Geometry: final body of the model. Coordinates: model frame, mm. Coordinates: 2 decimals unless noted, no trailing zeros. Order: outer loops, then holes, each group sorted by start corner. A loop starts at its lowest first (then second) coordinate and runs counter-clockwise, first axis right, second up. Notation, with made-up numbers: M -21.5,-3 L 14.5,-3 A16 ccw 14.5,26 Z; hole C 27.25,38 d4. An arc over 180 degrees is marked long. Write item = value, one per line.
from build123d import *

# Parameters (mm, degrees)
EXTRUDE_1_DEPTH     = 3
SKETCH_3_R          = 1.6
CUT_EXTRUDE_1_DEPTH = 92.836811791


with BuildPart() as part:
    # 草图1 → 凸台-拉伸1 (new body)
    with BuildSketch(Plane.XY):
        Polygon((0, 0), (0, 15), (13, 15), (30, 32), (30, 45), (50, 45), (50, 32), (67, 15), (80, 15), (80, 0), align=None)
    extrude(amount=EXTRUDE_1_DEPTH)

    # 草图3 → 切除-拉伸1 (cut, through all)
    with BuildSketch(Plane(origin=(0, 0, 0), x_dir=(-1, 0, 0), z_dir=(0, 0, -1))):
        with Locations((-46, 41)):
            Circle(SKETCH_3_R)
        with Locations((-34, 41)):
            Circle(SKETCH_3_R)
        with Locations((-46, 19)):
            Circle(SKETCH_3_R)
        with Locations((-34, 19)):
            Circle(SKETCH_3_R)
        with Locations((-34, 30)):
            Circle(SKETCH_3_R)
        with Locations((-46, 30)):
            Circle(SKETCH_3_R)
        with Locations((-74, 7)):
            Circle(SKETCH_3_R)
        with Locations((-66, 7)):
            Circle(SKETCH_3_R)
        with Locations((-58, 7)):
            Circle(SKETCH_3_R)
        with Locations((-50, 7)):
            Circle(SKETCH_3_R)
        with Locations((-6, 7)):
            Circle(SKETCH_3_R)
        with Locations((-14, 7)):
            Circle(SKETCH_3_R)
        with Locations((-22, 7)):
            Circle(SKETCH_3_R)
        with Locations((-29, 7)):
            Circle(SKETCH_3_R)
        with BuildLine():
            Line((-61.292893219, 16.464466094), (-55.636038969, 22.121320344))
            ThreePointArc((-55.636038969, 22.121320344), (-51.393398282, 22.121320344), (-51.393398282, 17.878679656))
            Line((-51.393398282, 17.878679656), (-57.050252532, 12.221825407))
            ThreePointArc((-57.050252532, 12.221825407), (-61.292893219, 12.221825407), (-61.292893219, 16.464466094))
        make_face()
        with BuildLine():
            Line((-22.949747468, 12.221825407), (-28.606601718, 17.878679656))
            ThreePointArc((-28.606601718, 17.878679656), (-28.606601718, 22.121320344), (-24.363961031, 22.121320344))
            Line((-24.363961031, 22.121320344), (-18.707106781, 16.464466094))
            ThreePointArc((-18.707106781, 16.464466094), (-18.707106781, 12.221825407), (-22.949747468, 12.221825407))
        make_face()
        with BuildLine():
            Line((-43, 5), (-43, 13))
            ThreePointArc((-43, 13), (-40, 16), (-37, 13))
            Line((-37, 13), (-37, 5))
            ThreePointArc((-37, 5), (-40, 2), (-43, 5))
        make_face()
    extrude(amount=-CUT_EXTRUDE_1_DEPTH, mode=Mode.SUBTRACT)


solid = part.part
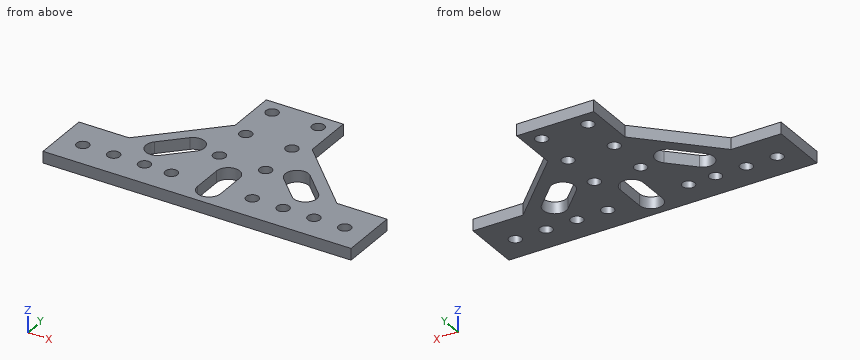
1) Line query: L1, parallel to Y at x = 46, z = 2; L2, parallel to Y at x = 40, z = 2.4; L3, parallel to X at y = 16.5, z = 0.3. Output: solid intervals per line, ascending.
Numbers:
L1 = 0 to 17.4, 20.6 to 28.4, 31.6 to 39.4, 42.6 to 45
L2 = 0 to 2, 16 to 45
L3 = 14.5 to 18.74, 27.23 to 52.77, 61.26 to 65.5
2) Section C-C, the plane x = 22. Return loops of the section in (y, z), and give its area (3 significant figures).
Numbers:
outline = M 0,0 L 5.4,0 L 5.4,3 L 0,3 Z; M 8.6,0 L 11.58,0 L 11.58,3 L 8.6,3 Z; M 19.76,0 L 24,0 L 24,3 L 19.76,3 Z
area = 37.9 mm²
3) Section A-A, the plane y = 41. Return loops of the section in (x, z), and give its area (3 significant figures).
Numbers:
outline = M 30,0 L 32.4,0 L 32.4,3 L 30,3 Z; M 35.6,0 L 44.4,0 L 44.4,3 L 35.6,3 Z; M 47.6,0 L 50,0 L 50,3 L 47.6,3 Z
area = 40.8 mm²
4) Section B-B, the plane x = 6. Return loops of the section in (y, z).
Numbers:
outline = M 0,0 L 5.4,0 L 5.4,3 L 0,3 Z; M 8.6,0 L 15,0 L 15,3 L 8.6,3 Z
5) Section D-D, the plane x = 14. Return loops of the section in (y, z), and give its area (3 significant figures).
Numbers:
outline = M 0,0 L 5.4,0 L 5.4,3 L 0,3 Z; M 8.6,0 L 16,0 L 16,3 L 8.6,3 Z
area = 38.4 mm²
6) Pin query (flat end, axial travel): pin 1 (3 mm diameter, centred on x = 50, y = 7, fed in from +Z); pin 2 (3.5 mm diameter, centred on x = 22, y = 7, fed in from +Z). Return the tip coordinate at first contact, or that it passes through.
Numbers:
pin_1 = through
pin_2 = 3
